Design review of the part built by this model. Coordinates are the model's own, in mm. A direction names the side the tool comes from. Coordinates: 2 decimals unless noted, no trailing zeros. Loops run counter-clockwise (first coordinate to the right, second up) from the corner with the lowest first, then second, coordinate; pieces in that order, holes last. Notation, with made-up numbers: (55, 73.5) -> (77, 73.5) arc R32 cw to (77, 105.5) -> close; hole circle Ø11 at (-22, -11). An arc over 180 degrees is marked (long way). Use a Markdown table: item, result. Add a question column.
Q1. For faces 5 (the face through (10.07, 15.6, 2.54)), 6 (the face through (-39.97, 1.35, 2.46)), 7 (the face through (14.5, 20, 2)), 8 (the face through (7.5, -23, 2)), 9 (the face through (-74.598, -13.338, 2.465)), list the 3-axis set-ups (+Z, -Z, +X, -X, +Y, -Y) from which the entire face can be reached by the end or side of a thin tool; tool diameter is ignored.
Q2. Take a section at C-C on x = -44. Write out the cut boundary in (y, z).
Q3. Take a section at A-A on y = 18. Write out the cut boundary in (x, z), plus the area to 3 significant figures.
Q4. Draft analysis for pull direction X (two halves, no side actions). For faces 1 (the face through (-65.35, -11.16, 2.46)), 2 (the face through (-2.5, 18, 2)), 3 (the face through (-22, -2, 0)), 4 (the face through (-57.223, -7.765, 2.465)), state which applies: pulls with the +X half, pulls with the -X half, needs draft (parallel to the pull), parting line crosses it, or undercut.
Q5. Take a section at B-B on y = 3. Write out the cut boundary in (x, z).
Q6. For probe 1 along Y at (x, z) = (5, 2.75); probe 2 along X at (y, z) = (13, 4.35); probe 3 along Y at (x, z) = (8, 2.4), list the stretches that pass through material, from the lowest coordinate up.
Q7. Clearance check with flat-ended pins moving along their axes: pin 1 Ø2 at (x, y) = (-55, 0) entering from -Z; pin 2 Ø10 at (x, y) = (-54, -10) entering from -Z; pin 3 Ø2 at (y, z) = (-12.5, 1) entering from +X; pin 4 Ø2.5 at (y, z) = (-11.5, 3.5) entering from -X. State where each tip first meets the part, or that it passes through.
from build123d import *

# Parameters (mm, degrees)
F0_W     = 5
F0_H     = 5
F1_DEPTH = 5
F2_R     = 2


with BuildPart() as f1:
    # F0 (on Top) → F1 (new body)
    with BuildSketch(Plane.XY):
        Polygon((2.5, 20), (2.5, 25), (-2.5, 25), (-2.5, 10), (-2.5, 4.868479), (-2.5, -25), (2.5, -25), (2.5, -20), align=None)
        Polygon((14.5, 25), (2.5, 25), (2.5, 20), (9.5, 20), (14.5, 20), align=None)
        Polygon((-2.5, 4.868479), (-2.5, 10), (-80.449605, -7.996084), (-79.32485, -12.867935), (-74.940185, -11.855655), (-65.683669, -9.71862), (-61.786189, -8.818816), (-52.529673, -6.681781), (-48.632193, -5.781976), (-39.375677, -3.644941), (-35.478197, -2.745137), (-26.221681, -0.608102), (-21.837016, 0.404178), align=None)
        with Locations((5, -22.5)):
            Rectangle(F0_W, F0_H)
        with Locations((12, 17.5)):
            Rectangle(F0_W, F0_H)
        Polygon((-20.262359, -6.416413), (-21.837016, 0.404178), (-26.221681, -0.608102), (-25.546828, -3.531212), (-25.809062, -4.618058), (-25.134209, -7.541168), align=None)
        Polygon((-74.940185, -11.855655), (-79.32485, -12.867935), (-77.750193, -19.688525), (-72.878342, -18.56377), (-73.553195, -15.64066), (-74.265331, -14.778765), align=None)
        Polygon((-34.803344, -5.668247), (-35.478197, -2.745137), (-39.375677, -3.644941), (-38.700824, -6.568052), (-38.963058, -7.654897), (-38.288205, -10.578007), (-33.416355, -9.453252), (-34.091208, -6.530142), align=None)
        Polygon((-61.786189, -8.818816), (-65.683669, -9.71862), (-65.008816, -12.64173), (-65.27105, -13.728576), (-64.596197, -16.651686), (-59.724346, -15.526931), (-60.399199, -12.60382), (-61.111336, -11.741926), align=None)
        Polygon((-47.95734, -8.705087), (-48.632193, -5.781976), (-52.529673, -6.681781), (-51.85482, -9.604891), (-52.117054, -10.691736), (-51.442201, -13.614847), (-46.57035, -12.490091), (-47.245204, -9.566981), align=None)
    extrude(amount=F1_DEPTH)

    # F2
    f2_edges = [f1.edges().sort_by_distance(p)[0] for p in [
        (-72.878342, -18.56377, 2.5),
        (-64.596197, -16.651686, 2.5),
        (-59.724346, -15.526931, 2.5),
        (-51.442201, -13.614847, 2.5),
        (-46.57035, -12.490091, 2.5),
        (-38.288205, -10.578007, 2.5),
        (-33.416355, -9.453252, 2.5),
        (-25.134209, -7.541168, 2.5),
        (-77.750193, -19.688525, 2.5),
        (-80.449605, -7.996084, 2.5),
        (-20.262359, -6.416413, 2.5),
        (9.5, 15, 2.5),
    ]]
    fillet(f2_edges, radius=F2_R)


solid = f1.part
Answer list:
| question | item | result |
|---|---|---|
| 1 | face 5 | +Z, -Z, -Y |
| 1 | face 6 | +Z, -Z, -X, +Y |
| 1 | face 7 | +Z, -Z, +X, +Y, -Y |
| 1 | face 8 | +Z, -Z, +X, -Y |
| 1 | face 9 | +Z, -Z |
| 2 | outline | (-4.71, 0) -> (0.42, 0) -> (0.42, 5) -> (-4.71, 5) -> close |
| 3 | outline | (-2.5, 0) -> (2.5, 0) -> (2.5, 5) -> (-2.5, 5) -> close; (9.5, 0) -> (14.5, 0) -> (14.5, 5) -> (9.5, 5) -> close |
| 3 | area | 50.0 mm² |
| 4 | face 1 | undercut |
| 4 | face 2 | pulls with the -X half |
| 4 | face 3 | needs draft |
| 4 | face 4 | undercut |
| 5 | outline | (-32.82, 0) -> (-10.59, 0) -> (-10.59, 5) -> (-32.82, 5) -> close; (-2.5, 0) -> (2.5, 0) -> (2.5, 5) -> (-2.5, 5) -> close |
| 6 | probe 1 | -25 to -20, 20 to 25 |
| 6 | probe 2 | -2.5 to 2.5 |
| 6 | probe 3 | 20 to 25 |
| 7 | pin 1 | through |
| 7 | pin 2 | z = 0 |
| 7 | pin 3 | x = 2.5 |
| 7 | pin 4 | x = -79.93 |
